```python
from build123d import *

# Parameters (mm, degrees)
F0_W     = 380
F0_H     = 235
F1_DEPTH = 10
F2_W     = 340
F2_H     = 185
F3_DEPTH = 3
F4_W     = 35
F4_H     = 75
F5_DEPTH = 1


with BuildPart() as f1:
    # F0 (on Front) → F1 (new body)
    with BuildSketch(Plane.XZ):
        Rectangle(F0_W, F0_H)
    extrude(amount=F1_DEPTH)

    # F2 (on face) → F3 (cut)
    with BuildSketch(Plane.XZ.offset(10)):
        with Locations((0, 5)):
            Rectangle(F2_W, F2_H)
    extrude(amount=-F3_DEPTH, mode=Mode.SUBTRACT)

    # F4 (on face) → F5 (cut)
    with BuildSketch(Plane(origin=(0, 0, 0), x_dir=(-1, 0, 0), z_dir=(0, 1, 0))):
        with Locations((-172.5, 60)):
            Rectangle(F4_W, F4_H)
        with Locations((-172.5, -50)):
            Rectangle(F4_W, F4_H)
        with Locations((172.5, -50)):
            Rectangle(F4_W, F4_H)
        with Locations((172.5, 60)):
            Rectangle(F4_W, F4_H)
    extrude(amount=-F5_DEPTH, mode=Mode.SUBTRACT)


solid = f1.part
```
The model under review builds one solid part; all positions refer to its coordinate system, in mm. A direction names the side the tool comes from. Coordinates: 2 decimals unless noted, no trailing zeros. Write each loop counter-clockwise with the first axis right and the second up, starting at its lowest first coordinate (ties: lowest second). Pieces come first, ordered by that corner, then holes. Notation, with made-up numbers: (48, 72) -> (75, 72) arc R28 ccw to (75, 101) -> close; hole circle Ø6 at (-31, 35). An arc over 180 degrees is marked (long way). One line per item, written item: value. Start each with the question number.
Q1. The part is to be moulded in two halves that separate along Z. For faces 4 (the face through (173, -1, -49)), 5 (the face through (-3, -5, -117.5)), 6 (the face through (-190, -5, -2)), say which applies: +Z half, -Z half, draft (parallel to the pull), parting line (faces both ways), or undercut.
Q2. Clearance check with flat-ended pins moving along their axes: P1, Ø17.5, axis at x = 177, z = 78, coming from the +Y side; P2, Ø0.5, axis at y = -0.5, z = 70, coming from the -X side; P3, Ø8, axis at x = 67, z = 6.5, coming from the -Y side. State where each tip first meets the part, or that it passes through.
Q3. For faces 1 (the face through (-2, -7, 6)), 2 (the face through (-172, -1, 61)), 3 (the face through (173, -1, 61)), list the 3-axis set-ups (+Z, -Z, +X, -X, +Y, -Y) from which the entire face can be reached by the end or side of a thin tool; tool diameter is ignored.
Q4. Add section B-B, the plane z = 55.5. Give the boundary of the cut face in (x, y), then the cut area to 3 significant figures.
Q5. Add section A-A, the plane x = -7.5. Give the boundary of the cut face in (y, z).
Q6. To check wall thickness, follow probe 1 along X at (y, z) = (-7.5, -85.5); probe 2 along Y at (x, z) = (68, 19); probe 3 along Z at (x, y) = (59, -9). State the ranges of each line that lie inside material, in increasing order.
Response:
1. face 4: undercut
1. face 5: -Z half
1. face 6: draft
2. P1: y = -1
2. P2: x = -155
2. P3: y = -7
3. face 1: -Y
3. face 2: -X, +Y
3. face 3: +X, +Y
4. outline: (-190, -10) -> (-170, -10) -> (-170, -7) -> (170, -7) -> (170, -10) -> (190, -10) -> (190, -1) -> (155, -1) -> (155, 0) -> (-155, 0) -> (-155, -1) -> (-190, -1) -> close
4. area: 2,710 mm²
5. outline: (-10, -117.5) -> (0, -117.5) -> (0, 117.5) -> (-10, 117.5) -> (-10, 97.5) -> (-7, 97.5) -> (-7, -87.5) -> (-10, -87.5) -> close
6. probe 1: -190 to -170, 170 to 190
6. probe 2: -7 to 0
6. probe 3: -117.5 to -87.5, 97.5 to 117.5
